from build123d import *

# Parameters (mm, degrees)
F0_W      = 25.4
F0_H      = 25.4
F1_DEPTH  = 101.6
F2_W      = 15.24
F2_H      = 15.24
F3_DEPTH  = 76.2
F6_START  = -3.175
F5_W      = 3.175
F5_H      = 15.24
F6_DEPTH  = 12.065
F4_R      = 2.15
F7_DEPTH  = 6.6675
F8_R      = 2.15
F9_DEPTH  = 6.6675
F10_W     = 1.27
F10_H     = 1.27
F12_DEPTH = 3.175
F11_W     = 1.27
F11_H     = 1.27
F13_DEPTH = 3.175
F14_W     = 12.7794421278
F14_H     = 4.0193349123
F15_DEPTH = 5.08
F16_W     = 25.4
F16_H     = 6.7783382893
F16_W_2   = 12.7794421278
F16_H_2   = 4.0193349123
F17_DEPTH = 5.08
F18_W     = 25.4
F18_H     = 6.7783382893
F19_DEPTH = 5.08
F20_R     = 2.15
F21_DEPTH = 5.08
F23_DEPTH = 25.4
F24_W     = 21.59
F24_H     = 2.35
F25_DEPTH = 77.47
F26_W     = 12.7794421278
F26_H     = 1.3284322977
F27_DEPTH = 5.08


with BuildPart() as f1:
    # F0 (on Top) → F1 (new body)
    with BuildSketch(Plane.XY):
        with Locations((12.7, 12.7)):
            Rectangle(F0_W, F0_H)
    extrude(amount=F1_DEPTH)

    # F2 (on face) → F3 (cut)
    with BuildSketch(Plane.XY.offset(101.6)):
        with Locations((12.7, 12.7)):
            Rectangle(F2_W, F2_H)
    extrude(amount=-F3_DEPTH, mode=Mode.SUBTRACT)

    # F5 (on face) → F6 (cut)
    with BuildSketch(Plane.XY.offset(25.4).offset(F6_START)):
        with Locations((17.145, 12.7)):
            Rectangle(F5_W, F5_H)
        with Locations((8.255, 12.7)):
            Rectangle(F5_W, F5_H)
    extrude(amount=-F6_DEPTH, mode=Mode.SUBTRACT)

    # F4 (on face) → F7 (cut, through all)
    with BuildSketch(Plane.YZ.offset(25.4)):
        with Locations((12.7, 12.7)):
            Circle(F4_R)
    extrude(amount=-F7_DEPTH, mode=Mode.SUBTRACT)

    # F8 (on face) → F9 (cut, through all)
    with BuildSketch(Plane(origin=(0, 0, 0), x_dir=(0, -1, 0), z_dir=(-1, 0, 0))):
        with Locations((-12.7, 12.7)):
            Circle(F8_R)
    extrude(amount=-F9_DEPTH, mode=Mode.SUBTRACT)

    # F10 (on face) → F12 (cut, through all)
    with BuildSketch(Plane.XY.offset(25.4)):
        with Locations((17.2085, 18.923)):
            Rectangle(F10_W, F10_H)
        with Locations((17.2085, 10.541)):
            Rectangle(F10_W, F10_H)
    extrude(amount=-F12_DEPTH, mode=Mode.SUBTRACT)

    # F11 (on face) → F13 (cut, through all)
    with BuildSketch(Plane.XY.offset(25.4)):
        with Locations((8.1467080774, 6.477)):
            Rectangle(F11_W, F11_H)
        with Locations((8.1467080774, 14.859)):
            Rectangle(F11_W, F11_H)
    extrude(amount=-F13_DEPTH, mode=Mode.SUBTRACT)

    # F14 (on face) → F15 (cut, through all)
    with BuildSketch(Plane(origin=(0, 0, 0), x_dir=(0, -1, 0), z_dir=(-1, 0, 0))):
        with Locations((-12.943365844, 98.2619002461)):
            Rectangle(F14_W, F14_H)
    extrude(amount=-F15_DEPTH, mode=Mode.SUBTRACT)

    # F16 (on face) → F17 (join)
    with BuildSketch(Plane(origin=(0, 0, 0), x_dir=(0, -1, 0), z_dir=(-1, 0, 0))):
        with Locations((-12.7, 98.2108308554)):
            Rectangle(F16_W, F16_H)
        with Locations((-12.943365844, 98.2619002461)):
            Rectangle(F16_W_2, F16_H_2, mode=Mode.SUBTRACT)
    extrude(amount=F17_DEPTH)

    # F18 (on face) → F19 (join)
    with BuildSketch(Plane(origin=(-5.08, 0, 0), x_dir=(0, -1, 0), z_dir=(-1, 0, 0))):
        with Locations((-12.7, 98.2108308554)):
            Rectangle(F18_W, F18_H)
    extrude(amount=F19_DEPTH)

    # F20 (on face) → F21 (cut)
    with BuildSketch(Plane(origin=(-10.16, 0, 0), x_dir=(0, -1, 0), z_dir=(-1, 0, 0))):
        with Locations((-12.7924755216, 98.2300043106)):
            Circle(F20_R)
    extrude(amount=-F21_DEPTH, mode=Mode.SUBTRACT)

    # F22 (on face) → F23 (join, through all)
    with BuildSketch(Plane.XZ):
        with BuildLine():
            ThreePointArc((-10.16, 94.8216617107), (-3.2465860676, 92.1186283067), (0, 85.4431986809))
            Line((0, 85.4431986809), (0, 94.8216617107))
            Line((0, 94.8216617107), (-10.16, 94.8216617107))
        make_face()
    extrude(amount=-F23_DEPTH)

    # F24 (on face) → F25 (cut)
    with BuildSketch(Plane.XY.offset(101.6)):
        with Locations((12.7, 16.859)):
            Rectangle(F24_W, F24_H)
        with Locations((12.7, 8.476)):
            Rectangle(F24_W, F24_H)
        with Locations((12.7, 12.731)):
            Rectangle(F24_W, F24_H)
    extrude(amount=-F25_DEPTH, mode=Mode.SUBTRACT)

    # F26 (on face) → F27 (cut)
    with BuildSketch(Plane.YZ.offset(5.08)):
        with Locations((12.943365844, 100.9357838511)):
            Rectangle(F26_W, F26_H)
    extrude(amount=-F27_DEPTH, mode=Mode.SUBTRACT)


solid = f1.part
Model file for the job. Use its own axes, mm. A direction names the side the tool comes from. Coordinates: 2 decimals unless noted, no trailing zeros. Loops run counter-clockwise (first coordinate to the right, second up) from the corner with the lowest first, then second, coordinate; pieces in that order, holes last. Notation, with made-up numbers: (84.25, 49.5) -> (121.25, 49.5) arc R23 ccw to (121.25, 75.5) -> close; hole circle Ø2 at (87.5, -27.75). An arc over 180 degrees is marked (long way). Use one line per item in the form item = value. Start each with the question number.
(1) Pull direction X, two halves, no side cores. Call faces 6 (the flat face through (-10.16, 13, 101)), 7 (the flat face through (21, 9.651, 63)), 8 (the flat face through (11, 25.4, 52)): pulls with the +X half, pulls with the -X half, needs draft (parallel to the pull), parting line crosses it, or undercut.
(2) Probe probe 1 along Y at (x, z) = (21, 28); probe 2 along Z at (x, y) = (9.5, 11.5) (3 decimals); probe 3 along Z at (x, y) = (4.5, 12.7). List the from-to ranges inside material, lowest first. Write a range as from..to.
(3) Cut at B-B on x = 22. Give the cut face in (y, z), and give its area (3 significant figures).
(4) Tool access for faces 1 (the flat face through (13, 13, 0)), 2 (the cylindrical face through (22.11, 12.42, 14.83)), 3 (the flat face through (25.4, 13, 50)), 4 (the flat face through (5.08, 11, 61)), 5 (the flat face through (17, 5.08, 16)): list every direction of +Z, -Z, +X, -X, +Y, -Y with a clear straight run to the whole face (end or side of a thin tool).
(5) Flat gauge pins, fed straight in: pin 1 (1.4 mm diameter, centred on y = 10.5, z = 23.5, fed in from -X); pin 2 (2.5 mm diameter, centred on x = 15.5, y = 18.5, fed in from +Z). Where does each tip first touch, or does it go through?
(6) Cut at C-C on y = 16.75. Give the cut face in (x, z) (1 decimal).
(7) Cut at D-D on z = 12.7. Give the cut face in (x, y).
Values:
q1.face_6 = pulls with the -X half
q1.face_7 = undercut
q1.face_8 = needs draft
q2.probe_1 = 0..7.3, 9.65..11.56, 13.91..15.68, 18.03..25.4
q2.probe_2 = 0..10.16, 22.225..25.4
q2.probe_3 = 0..10.55, 14.85..24.13
q3.outline = (0, 0) -> (25.4, 0) -> (25.4, 101.6) -> (18.03, 101.6) -> (18.03, 24.13) -> (15.68, 24.13) -> (15.68, 101.6) -> (13.91, 101.6) -> (13.91, 24.13) -> (11.56, 24.13) -> (11.56, 101.6) -> (9.65, 101.6) -> (9.65, 24.13) -> (7.3, 24.13) -> (7.3, 101.6) -> (0, 101.6) -> close; hole circle Ø4.3 at (12.7, 12.7)
q3.area = 2,020 mm2
q4.face_1 = -Z, +X, -X, +Y, -Y
q4.face_2 = +X
q4.face_3 = +Z, -Z, +X, +Y, -Y
q4.face_4 = +Z
q4.face_5 = none
q5.pin_1 = 0
q5.pin_2 = 25.4
q6.outline = (-10.2, 94.8) arc R10.2 cw to (0, 85.4) -> (0, 0) -> (25.4, 0) -> (25.4, 101.6) -> (23.5, 101.6) -> (23.5, 24.1) -> (1.9, 24.1) -> (1.9, 96.3) -> (-5.1, 96.3) -> (-5.1, 100.3) -> (0, 100.3) -> (0, 101.6) -> (-10.2, 101.6) -> close; hole (6.7, 10.2) -> (9.8, 10.2) -> (9.8, 22.2) -> (6.7, 22.2) -> close; hole (15.6, 10.2) -> (18.7, 10.2) -> (18.7, 22.2) -> (15.6, 22.2) -> close
q7.outline = (0, 0) -> (25.4, 0) -> (25.4, 10.55) -> (18.73, 10.55) -> (18.73, 5.08) -> (15.56, 5.08) -> (15.56, 20.32) -> (18.73, 20.32) -> (18.73, 14.85) -> (25.4, 14.85) -> (25.4, 25.4) -> (0, 25.4) -> (0, 14.85) -> (6.67, 14.85) -> (6.67, 20.32) -> (9.84, 20.32) -> (9.84, 5.08) -> (6.67, 5.08) -> (6.67, 10.55) -> (0, 10.55) -> close
